Check sheet for the modelled part. Datum: model origin and axes. Units: mm. Face numbers are marked on the shaded views. A direction names the side the tool comes from. Coordinates: 2 decimals unless noted, no trailing zeros. Write each loop counter-clockwise with the first axis right and the second up, starting at its lowest first coordinate (ties: lowest second). Pieces come first, ordered by that corner, then holes. Notation, with made-up numbers: (-33, 65) - (-13, 65) arc R35 ccw to (-13, 103) - close; hole circle Ø4 at (46.5, 29). An arc over 180 degrees is marked (long way). Answer as CSV lines item,"result". Start each with the question number.
from build123d import *
from build123d.topology import SkipClean

# Parameters (mm, degrees)
SKETCH2_R           = 16.5
SKETCH2_R_2         = 14
SKETCH2_R_3         = 2
BOSS_EXTRUDE1_DEPTH = 12
BOSS_EXTRUDE2_START = 5
SKETCH3_R           = 2
SKETCH3_R_2         = 16.5
BOSS_EXTRUDE2_DEPTH = 5


with BuildPart() as part:
    # Sketch2 → Boss-Extrude1 (new body)
    with BuildSketch(Plane.XY):
        with BuildLine():
            Line((35, 53.138686131), (35, -126.861313869))
            ThreePointArc((35, -126.861313869), (0, -161.861313869), (-35, -126.861313869))
            Line((-35, -126.861313869), (-35, 53.138686131))
            ThreePointArc((-35, 53.138686131), (0, 88.138686131), (35, 53.138686131))
        make_face()
        with Locations((0, 53.138686131)):
            Circle(SKETCH2_R, mode=Mode.SUBTRACT)
        with Locations((0, -126.861313869)):
            Circle(SKETCH2_R_2, mode=Mode.SUBTRACT)
        with Locations((0, 78.138686131)):
            Circle(SKETCH2_R_3, mode=Mode.SUBTRACT)
        with Locations((-25, 53.138686131)):
            Circle(SKETCH2_R_3, mode=Mode.SUBTRACT)
        with Locations((0, 28.138686131)):
            Circle(SKETCH2_R_3, mode=Mode.SUBTRACT)
        with Locations((25, 53.138686131)):
            Circle(SKETCH2_R_3, mode=Mode.SUBTRACT)
    extrude(amount=BOSS_EXTRUDE1_DEPTH)

    # Sketch3 → Boss-Extrude2 (add)
    with SkipClean():  # the faces are left unmerged after this step: merging them gives an invalid solid
        with BuildSketch(Plane(origin=(0, 0, 0), x_dir=(-1, 0, 0), z_dir=(0, 0, -1)).offset(BOSS_EXTRUDE2_START)):
            with BuildLine():
                ThreePointArc((35, 53.138686131), (0, 88.138686131), (-35, 53.138686131))
                ThreePointArc((-35, 53.138686131), (0, 18.138686131), (35, 53.138686131))
            make_face()
            with Locations((-25, 53.138686131)):
                Circle(SKETCH3_R, mode=Mode.SUBTRACT)
            with Locations((0, 28.138686131)):
                Circle(SKETCH3_R, mode=Mode.SUBTRACT)
            with Locations((0, 53.138686131)):
                Circle(SKETCH3_R_2, mode=Mode.SUBTRACT)
            with Locations((0, 78.138686131)):
                Circle(SKETCH3_R, mode=Mode.SUBTRACT)
            with Locations((25, 53.138686131)):
                Circle(SKETCH3_R, mode=Mode.SUBTRACT)
        extrude(amount=-BOSS_EXTRUDE2_DEPTH)


solid = part.part
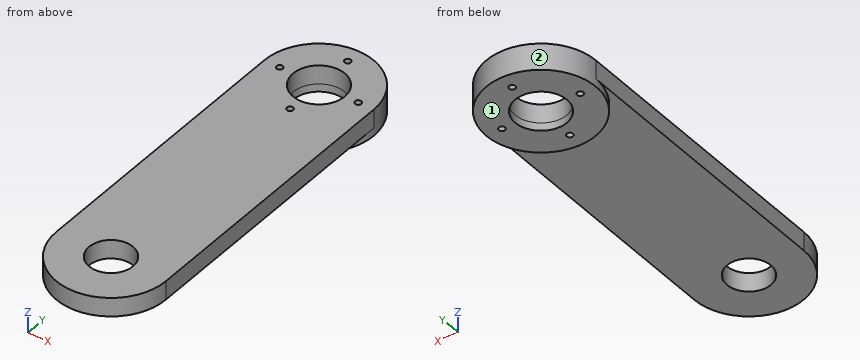
(1) Material ranges on probe 1 along Y at (x, z) = (0, 4.25); probe 2 along Y at (x, z) = (-10.5, 4.25); probe 3 along Z at (x, y) = (16.5, 3.5), recorded low to high. Write a range as from..to.
(2) Cross-section at C-C on y = -47. Record the boundary of the cut face in (x, z).
(3) Tool access check on the marked faces 1 and 2. Record the directions out of +Z, -Z, +X, -X, +Y, -Y that give a thin tool (end or side, any length) a straight path to the whole face; none if there is none.
(4) Cross-section at B-B on z = 8.5. Record the boundary of the cut face in (x, y).
(5) Go/stop test with flat-tipped pins: P1, Ø6, axis at x = 23, z = 7, coming from the +Y side; P2, Ø1, axis at x = -18.5, z = 3, coming from the -Y side; P3, Ø2, axis at x = 22, z = 0.5, coming from the -Y side. Record where each tip stops, or that it passes through.
(6) Cross-section at A-A on x = 8. Record the boundary of the cut face in (y, z), plus the area to 3 significant figures.
Checked values:
1,probe 1,"-161.86..-140.86, -112.86..26.14, 30.14..36.64, 69.64..76.14, 80.14..88.14"
1,probe 2,"-160.25..-136.12, -117.6..40.41, 65.87..86.53"
1,probe 3,"0..12"
2,outline,"(-35, 0) - (35, 0) - (35, 12) - (-35, 12) - close"
3,face 1,"-Z, +X, -X, +Y, -Y"
3,face 2,"-Z"
4,outline,"(-35, -126.86) arc R35 ccw to (35, -126.86) - (35, 53.14) arc R35 ccw to (-35, 53.14) - close; hole circle Ø4 at (-25, 53.14); hole circle Ø33 at (0, 53.14); hole circle Ø28 at (0, -126.86); hole circle Ø4 at (0, 28.14); hole circle Ø4 at (0, 78.14); hole circle Ø4 at (25, 53.14)"
5,P1,"y = 81.86"
5,P2,"y = -156.88"
5,P3,"y = -154.86"
6,outline,"(-160.93, 0) - (-138.35, 0) - (-138.35, 12) - (-160.93, 12) - close; (-115.37, 0) - (19.07, 0) - (19.07, -5) - (38.71, -5) - (38.71, 12) - (-115.37, 12) - close; (67.57, -5) - (87.21, -5) - (87.21, 12) - (67.57, 12) - close"
6,area,"2,550 mm^2"
